CAD build for the part. Positions are in the model's coordinates, mm. A direction names the side the tool comes from. Round coordinates to 2 decimals unless told otherwise and drop trailing zeros. Order: outer loops, then holes, each group sorted by start corner. A loop starts at its lowest first (then second) coordinate and runs counter-clockwise, first axis right, second up. Notation, with made-up numbers: (-6.5, 56) -> (8.5, 56) arc R11 ccw to (8.5, 64) -> close; hole circle Ø2 at (27.25, 86). An arc over 180 degrees is marked (long way). Return JSON: item names as keys, results as strings. Group by question number.
Q1. Cut at A-A (z = 0). Write the cut outline in (x, y).
Q2. Probe line 1 along Z through (x, y) = (0, 1.2); line 2 along Z through (x, y) = (0, 2.35); line 3 along X through (y, z) = (0.7, 0). List the from-to ranges inside material, lowest first.
Q3. Mould opens along X. For faces 1 (the flat face through (15, 1.5, 4)), 2 (the flat face through (-64.1, 2, 1)), 3 (the flat face through (64.1, 2, 1)) say: +X half, -X half, draft (parallel to the pull), parting line (faces both ways), or undercut.
Q4. Which spindle directions (+Z, -Z, +X, -X, +Y, -Y) get a long thin tool onto all of the face, cutting with end or side? Do faces 4 (the cylindrical face through (2.343, 2.26, 17.847)), 5 (the cylindrical face through (-12.1, 1.01, 9.28)). Say none if no direction does.
Q5. Cut at B-B (x = 0). Write the cut outline in (y, z), then the cut area to 3 significant figures.
from build123d import *

# Parameters (mm, degrees)
SKETCH1_W      = 128.2
SKETCH1_H      = 86
EXTRUDE1_DEPTH = 5
SKETCH4_R      = 18
EXTRUDE4_DEPTH = 3.5
SKETCH6_R      = 15.25
EXTRUDE6_DEPTH = 2.5
CHAMFER5_SIZE  = 0.5
CHAMFER6_SIZE  = 2
CHAMFER7_SIZE  = 0.25


with BuildPart() as part:
    # Sketch1 → Extrude1 (new body)
    with BuildSketch(Plane(origin=(0, 0, 0), x_dir=(1, 0, 0), z_dir=(0, 1, 0))):
        Rectangle(SKETCH1_W, SKETCH1_H)
    extrude(amount=EXTRUDE1_DEPTH)

    # Sketch4 → Extrude4 (cut)
    with BuildSketch(Plane(origin=(0, 5, 0), x_dir=(-1, 0, 0), z_dir=(0, 1, 0))):
        Circle(SKETCH4_R)
    extrude(amount=-EXTRUDE4_DEPTH, mode=Mode.SUBTRACT)

    # Sketch6 → Extrude6 (cut, through all)
    with BuildSketch(Plane(origin=(0, 1.5, 0), x_dir=(1, 0, 0), z_dir=(0, 1, 0))):
        Circle(SKETCH6_R)
    extrude(amount=-EXTRUDE6_DEPTH, mode=Mode.SUBTRACT)

    # Chamfer5
    chamfer5_edges = [part.edges().sort_by_distance(p)[0] for p in [
        (-15.25, 0, 0),
    ]]
    chamfer(chamfer5_edges, length=CHAMFER5_SIZE)

    # Chamfer6
    chamfer6_edges = [part.edges().sort_by_distance(p)[0] for p in [
        (18, 5, 0),
    ]]
    chamfer(chamfer6_edges, length=CHAMFER6_SIZE)

    # Chamfer7
    chamfer7_edges = [part.edges().sort_by_distance(p)[0] for p in [
        (-64.1, 5, 0),
        (0, 5, 43),
        (64.1, 5, 0),
        (0, 0, 43),
        (-64.1, 0, 0),
        (0, 0, -43),
        (64.1, 0, 0),
        (0, 5, -43),
        (64.1, 2.5, 43),
        (-64.1, 2.5, 43),
        (-64.1, 2.5, -43),
        (64.1, 2.5, -43),
    ]]
    chamfer(chamfer7_edges, length=CHAMFER7_SIZE)


solid = part.part
Solution:
{
 "1": {"outline": "(-64.1, 0.25) -> (-63.85, 0) -> (-15.75, 0) -> (-15.25, 0.5) -> (-15.25, 1.5) -> (-18, 1.5) -> (-18, 3) -> (-20, 5) -> (-63.85, 5) -> (-64.1, 4.75) -> close; (15.25, 0.5) -> (15.75, 0) -> (63.85, 0) -> (64.1, 0.25) -> (64.1, 4.75) -> (63.85, 5) -> (20, 5) -> (18, 3) -> (18, 1.5) -> (15.25, 1.5) -> close"},
 "2": {"line 1": "z = -43 to -15.25, 15.25 to 43", "line 2": "z = -43 to -18, 18 to 43", "line 3": "x = -64.1 to -15.25, 15.25 to 64.1"},
 "3": {"face 1": "undercut", "face 2": "-X half", "face 3": "+X half"},
 "4": {"face 4": "+Y", "face 5": "+Y, -Y"},
 "5": {"outline": "(0, -42.75) -> (0.25, -43) -> (4.75, -43) -> (5, -42.75) -> (5, -20) -> (3, -18) -> (1.5, -18) -> (1.5, -15.25) -> (0.5, -15.25) -> (0, -15.75) -> close; (0, 15.75) -> (0.5, 15.25) -> (1.5, 15.25) -> (1.5, 18) -> (3, 18) -> (5, 20) -> (5, 42.75) -> (4.75, 43) -> (0.25, 43) -> (0, 42.75) -> close", "area": "254 mm²"}
}
